```python
from build123d import *

# Parameters (mm, degrees)
SKETCH1_W           = 35
SKETCH1_H           = 27
BOSS_EXTRUDE1_DEPTH = 14
SKETCH2_R           = 1.75
CUT_EXTRUDE1_DEPTH  = 14
SKETCH9_R           = 3
CUT_EXTRUDE7_DEPTH  = 10
SKETCH10_W          = 35
SKETCH10_H          = 4.5
BOSS_EXTRUDE2_DEPTH = 4
SKETCH11_W          = 35
SKETCH11_H          = 2.5
CUT_EXTRUDE8_DEPTH  = 6
BOSS_EXTRUDE3_DEPTH = 2.5
BOSS_EXTRUDE4_DEPTH = 2.5
SKETCH14_W          = 5
SKETCH14_H          = 6
BOSS_EXTRUDE5_DEPTH = 1.5
SKETCH15_W          = 40
SKETCH15_H          = 2.5
CUT_EXTRUDE9_DEPTH  = 7
SKETCH16_W          = 5
SKETCH16_H          = 7
BOSS_EXTRUDE6_DEPTH = 1.5


with BuildPart() as part:
    # Sketch1 → Boss-Extrude1 (new body)
    with BuildSketch(Plane(origin=(0, 0, 0), x_dir=(1, 0, 0), z_dir=(0, 1, 0))):
        Rectangle(SKETCH1_W, SKETCH1_H)
    extrude(amount=BOSS_EXTRUDE1_DEPTH)

    # Sketch2 → Cut-Extrude1 (cut)
    with BuildSketch(Plane(origin=(0, 14, 0), x_dir=(1, 0, 0), z_dir=(0, 1, 0))):
        with Locations(Location((7.5, 10, 0), (0, 0, 270))):
            Circle(SKETCH2_R)
        with Locations(Location((-7.5, -10, 0), (0, 0, 270))):
            Circle(SKETCH2_R)
    extrude(amount=-CUT_EXTRUDE1_DEPTH, mode=Mode.SUBTRACT)

    # Sketch9 → Cut-Extrude7 (cut)
    with BuildSketch(Plane(origin=(0, 14, 0), x_dir=(1, 0, 0), z_dir=(0, 1, 0))):
        with Locations(Location((7.5, 10, 0), (0, 0, 270))):
            Circle(SKETCH9_R)
        with Locations(Location((-7.5, -10, 0), (0, 0, 270))):
            Circle(SKETCH9_R)
    extrude(amount=-CUT_EXTRUDE7_DEPTH, mode=Mode.SUBTRACT)

    # Sketch10 → Boss-Extrude2 (add)
    with BuildSketch(Plane.XZ):
        Rectangle(SKETCH10_W, SKETCH10_H)
    extrude(amount=BOSS_EXTRUDE2_DEPTH)

    # Sketch11 → Cut-Extrude8 (cut)
    with BuildSketch(Plane.XZ.offset(4)):
        Rectangle(SKETCH11_W, SKETCH11_H)
    extrude(amount=-CUT_EXTRUDE8_DEPTH, mode=Mode.SUBTRACT)

    # Sketch12 → Boss-Extrude3 (add)
    with BuildSketch(Plane.ZY.offset(17.5)):
        Polygon((-2.25, -4), (-2.25, 0), (-2.25, 14), (2.25, 14), (2.25, 0), (2.25, -4), (1.25, -4), (1.25, 2), (-1.25, 2), (-1.25, -4), align=None)
    extrude(amount=BOSS_EXTRUDE3_DEPTH)

    # Sketch13 → Boss-Extrude4 (add)
    with BuildSketch(Plane(origin=(17.5, 0, 0), x_dir=(0, 0, -1), z_dir=(1, 0, 0))):
        Polygon((2.25, -4), (2.25, 0), (2.25, 14), (-2.25, 14), (-2.25, 0), (-2.25, -4), (-1.25, -4), (-1.25, 2), (1.25, 2), (1.25, -4), align=None)
    extrude(amount=BOSS_EXTRUDE4_DEPTH)

    # Sketch14 → Boss-Extrude5 (add)
    with BuildSketch(Plane(origin=(0, 0, 1.25), x_dir=(-1, 0, 0), z_dir=(0, 0, -1))):
        with Locations((-17.5, -1)):
            Rectangle(SKETCH14_W, SKETCH14_H)
        with Locations((17.5, -1)):
            Rectangle(SKETCH14_W, SKETCH14_H)
    extrude(amount=BOSS_EXTRUDE5_DEPTH)

    # Sketch15 → Cut-Extrude9 (cut)
    with BuildSketch(Plane(origin=(0, 14, 0), x_dir=(1, 0, 0), z_dir=(0, 1, 0))):
        Rectangle(SKETCH15_W, SKETCH15_H)
    extrude(amount=-CUT_EXTRUDE9_DEPTH, mode=Mode.SUBTRACT)

    # Sketch16 → Boss-Extrude6 (add)
    with BuildSketch(Plane(origin=(0, 0, 1.25), x_dir=(-1, 0, 0), z_dir=(0, 0, -1))):
        with Locations((-17.5, 10.5)):
            Rectangle(SKETCH16_W, SKETCH16_H)
        with Locations((17.5, 10.5)):
            Rectangle(SKETCH16_W, SKETCH16_H)
    extrude(amount=BOSS_EXTRUDE6_DEPTH)


solid = part.part
```
Verification items for the finished model (mm, model axes). A direction names the side the tool comes from. Round coordinates to 2 decimals unless told otherwise and drop trailing zeros. Write each loop counter-clockwise with the first axis right and the second up, starting at its lowest first coordinate (ties: lowest second). Pieces come first, ordered by that corner, then holes. Notation, with made-up numbers: (5, 77) -> (28, 77) arc R18 ccw to (28, 100) -> close; hole circle Ø5 at (-7.75, 23). An arc over 180 degrees is marked (long way). Write each question's results on one line, items separated by ' | '. Start each with the question number.
1. Cross-section at C-C (z = -11.25). Enter the section's corners in (x, y).
2. Cross-section at D-D (x = 13). Enter the section's corners in (y, z), then the cut area to 4 significant figures.
3. Set-up check for faces 4 (the flat face through (15, -1, 1)), 5 (the flat face through (0, 7, 13.5)), 6 (the cylindrical face through (7.6, 9.1, -13)), 7 (the flat face through (-17, 11, -0.25)), 8 (the flat face through (18, -1, -0.25)): record each of +Z, -Z, +X, -X, +Y, -Y from which the full face is reachable in a straight line by a thin tool's end or side.
4. Material ranges on probe 1 along X at (y, z) = (2.85, -10); probe 2 along X at (y, z) = (10, 10); probe 3 along Z at (x, y) = (18.5, 0), recorded low to high. Write a range as from..to.
5. Draft check along X on faces 1 (the flat face through (17.5, 7, -8)), 2 (the flat face through (18, 11, -0.25)), 3 (the flat face through (15, 10, 1)). Enter one of: +X half, -X half, draft (parallel to the pull), parting line (faces both ways), or undercut.
6. Cross-section at B-B (x = -7.5). Enter the section's corners in (y, z).
7. Depth check by flat-ended pin: P1, Ø3, axis at x = -7.5, z = 9.5, coming from the +Y side; P2, Ø6, axis at y = 5.5, z = -8, coming from the +X side; P3, Ø3.5, axis at y = 7, z = 7, coming from the -X side. Enter the tip coordinate at first touch or a pass-through.
8. Cross-section at A-A (y = 0.5). Enter the section's corners in (x, z).
Solutions:
1) outline: (-17.5, 0) -> (6.28, 0) -> (6.28, 4) -> (4.77, 4) -> (4.77, 14) -> (-17.5, 14) -> close; (8.72, 0) -> (17.5, 0) -> (17.5, 14) -> (10.23, 14) -> (10.23, 4) -> (8.72, 4) -> close
2) outline: (-4, -2.25) -> (0, -2.25) -> (0, -13.5) -> (14, -13.5) -> (14, -1.25) -> (7, -1.25) -> (7, 1.25) -> (14, 1.25) -> (14, 13.5) -> (0, 13.5) -> (0, 2.25) -> (-4, 2.25) -> (-4, 1.25) -> (2, 1.25) -> (2, -1.25) -> (-4, -1.25) -> close | area: 363.5 mm2
3) face 4: -Y | face 5: +Z, +X, -X, +Y, -Y | face 6: +Y | face 7: +X, -X, +Y | face 8: +X, -X, -Y
4) probe 1: x = -17.5..5.75, 9.25..17.5 | probe 2: x = -17.5..-10.5, -4.5..17.5 | probe 3: z = -2.25..-1.25, -0.25..2.25
5) face 1: +X half | face 2: draft | face 3: undercut
6) outline: (-4, -2.25) -> (0, -2.25) -> (0, -13.5) -> (14, -13.5) -> (14, -1.25) -> (7, -1.25) -> (7, 1.25) -> (14, 1.25) -> (14, 7) -> (4, 7) -> (4, 8.25) -> (0, 8.25) -> (0, 2.25) -> (-4, 2.25) -> (-4, 1.25) -> (2, 1.25) -> (2, -1.25) -> (-4, -1.25) -> close; (0, 11.75) -> (4, 11.75) -> (4, 13) -> (14, 13) -> (14, 13.5) -> (0, 13.5) -> close
7) P1: stops at y = 4 | P2: stops at x = 17.5 | P3: stops at x = -17.5
8) outline: (-20, -2.25) -> (-17.5, -2.25) -> (-17.5, -13.5) -> (17.5, -13.5) -> (17.5, -2.25) -> (20, -2.25) -> (20, -1.25) -> (-20, -1.25) -> close; (-20, -0.25) -> (-15, -0.25) -> (-15, 1.25) -> (15, 1.25) -> (15, -0.25) -> (20, -0.25) -> (20, 2.25) -> (17.5, 2.25) -> (17.5, 13.5) -> (-17.5, 13.5) -> (-17.5, 2.25) -> (-20, 2.25) -> close; hole circle Ø3.5 at (-7.5, 10); hole circle Ø3.5 at (7.5, -10)
